Source: CAD feature listing. Evaluate the final solid. Frame: model axes, mm. A direction names the side the tool comes from. Round coordinates to 2 decimals unless told otherwise and drop trailing zeros. Order: outer loops, then holes, each group sorted by start corner. A loop starts at its lowest first (then second) coordinate and runs counter-clockwise, first axis right, second up. Notation, with made-up numbers: (-39.75, -16.5) - (19.25, -16.5) arc R20 cw to (19.25, 8.5) - close; hole circle Ø1 at (65, 51). An arc over 180 degrees is marked (long way). Put each result on its own line as item: value. Start each with the question number.
1) Line query: probe 1 along X at (y, z) = (2, -1); probe 2 along Z at (x, y) = (7, -2.5); probe 3 along X at (y, z) = (-1.5, 8.5). Output: solid intervals per line, ascending. Write a range as [from, to].
2) Access query for faces 4 (the face through (8, 1.95, 8)), 5 (the face through (6.3, 0, 8)), 6 (the face through (10.1, 0, 8)), 7 (the face through (8, -1, 11)). Directions: +Z, -Z, +X, -X, +Y, -Y. A direction counts if a zero-diameter tool reaches every point of the face in a straight line with its end or side. Return the directions, or none.
3) Section A-A on y = -1.25. Output: boundary loops of the cut face in (x, z), then the cut area to 3 significant figures.
4) Mould query, pull axis Y, two halves, no side actions, for faces 1 (the face through (6.144, 0.231, -1.775)), 2 (the face through (8, -1.95, 8)), 3 (the face through (11, 0, -3.6)). Classes: +Y half, -Y half, draft (parallel to the pull), parting line (faces both ways), or undercut.
5) Section D-D on x = 10.7. Output: boundary loops of the cut face in (y, z), then the cut area to 3 significant figures.
6) Section C-C on z = 9. Output: boundary loops of the cut face in (x, y).
7) Contact query for flat-ended pins moving along their axis: P1, Ø0.9, axis at x = 8, z = 11.5, coming from the +Y side; P2, Ø0.7, axis at x = 8, z = 8, coming from the -Y side; P3, Ø1, axis at y = -0.5, z = 11, coming from the +X side. Output: stop coordinate, or through.
8) Section B-B on x = 7.75. Output: boundary loops of the cut face in (y, z).
```python
from build123d import *

# Parameters (mm, degrees)
SKETCH069_W             = 7
SKETCH069_H             = 7
PAD039_DEPTH            = 7.1
SKETCH070_R             = 0.5
PAD040_DEPTH            = 3.6
SKETCH071_W             = 3.9
SKETCH071_H             = 3.8
PAD041_DEPTH            = 9.4
SKETCH072_W             = 2
SKETCH072_H             = 3
PAD042_DEPTH            = 12.3
BODY057_PLACEMENT_ANGLE = 90


with BuildPart() as part:
    # Sketch069 → Pad039 (new body)
    with BuildSketch(Plane.XY):
        Rectangle(SKETCH069_W, SKETCH069_H)
    extrude(amount=PAD039_DEPTH)

    # Sketch070 → Pad040 (join)
    with BuildSketch(Plane.XY):
        with Locations((0, 2.5)):
            Circle(SKETCH070_R)
        with Locations((0, -2.5)):
            Circle(SKETCH070_R)
        with Locations((2, 2.5)):
            Circle(SKETCH070_R)
        with Locations((-2, 2.5)):
            Circle(SKETCH070_R)
        with Locations((-2, -2.5)):
            Circle(SKETCH070_R)
        with Locations((2, -2.5)):
            Circle(SKETCH070_R)
    extrude(amount=-PAD040_DEPTH)

    # Sketch071 → Pad041 (join)
    with BuildSketch(Plane.XY):
        Rectangle(SKETCH071_W, SKETCH071_H)
    extrude(amount=PAD041_DEPTH)

    # Sketch072 → Pad042 (join)
    with BuildSketch(Plane.XY):
        Rectangle(SKETCH072_W, SKETCH072_H)
    extrude(amount=PAD042_DEPTH)


with BuildPart() as part_1:
    # Body057 placement: moved
    add(part.part.moved(Location((8.2, 0, 0))).rotate(Axis((8.2, 0, 0), (0, 0, 1)), BODY057_PLACEMENT_ANGLE))


solid = part_1.part
```
Answer sheet:
1. probe 1: [5.2, 6.2], [10.2, 11.2]
1. probe 2: [0, 7.1]
1. probe 3: [6.3, 10.1]
2. face 4: +Z, +X, -X, +Y
2. face 5: +Z, -X, +Y, -Y
2. face 6: +Z, +X, +Y, -Y
2. face 7: +Z, +X, -X, -Y
3. outline: (4.7, 0) - (11.7, 0) - (11.7, 7.1) - (10.1, 7.1) - (10.1, 9.4) - (6.3, 9.4) - (6.3, 7.1) - (4.7, 7.1) - close
3. area: 58.4 mm^2
4. face 1: undercut
4. face 2: -Y half
4. face 3: draft
5. outline: (-3.5, 0) - (-2.5, 0) - (-2.5, -3.6) - (-1.5, -3.6) - (-1.5, 0) - (-0.5, 0) - (-0.5, -3.6) - (0.5, -3.6) - (0.5, 0) - (1.5, 0) - (1.5, -3.6) - (2.5, -3.6) - (2.5, 0) - (3.5, 0) - (3.5, 7.1) - (-3.5, 7.1) - close
5. area: 60.5 mm^2
6. outline: (6.3, -1.95) - (10.1, -1.95) - (10.1, 1.95) - (6.3, 1.95) - close
7. P1: y = 1
7. P2: y = -1.95
7. P3: x = 9.7
8. outline: (-3.5, 0) - (3.5, 0) - (3.5, 7.1) - (1.95, 7.1) - (1.95, 9.4) - (1, 9.4) - (1, 12.3) - (-1, 12.3) - (-1, 9.4) - (-1.95, 9.4) - (-1.95, 7.1) - (-3.5, 7.1) - close
